from build123d import *

# Parameters (mm, degrees)
SKETCH1_R           = 4
BOSS_EXTRUDE1_DEPTH = 15
SKETCH2_R           = 6
BOSS_EXTRUDE2_DEPTH = 1
DOME1_FACE_RADIUS   = 6
DOME1_HEIGHT        = 6
SKETCH3_W           = 2
SKETCH3_H           = 12.932996947
CUT_EXTRUDE2_DEPTH  = 5


with BuildPart() as part:
    # Sketch1 → Boss-Extrude1 (new body)
    with BuildSketch(Plane.XY):
        Circle(SKETCH1_R)
    extrude(amount=BOSS_EXTRUDE1_DEPTH)

    # Sketch2 → Boss-Extrude2 (add)
    with BuildSketch(Plane.XY.offset(15)):
        Circle(SKETCH2_R)
    extrude(amount=BOSS_EXTRUDE2_DEPTH)

    # Dome1: a dome of height H over a round flat face of radius A is a cap of a sphere of radius (A * A + H * H) / (2 * H)
    dome1_r = (DOME1_FACE_RADIUS * DOME1_FACE_RADIUS + DOME1_HEIGHT * DOME1_HEIGHT) / (2 * DOME1_HEIGHT)
    dome1_base = Plane((0, 0, 16), z_dir=(0, 0, 1))
    with Locations(dome1_base.offset(DOME1_HEIGHT - dome1_r)):
        dome1_ball = Sphere(dome1_r, mode=Mode.PRIVATE)
    add(split(dome1_ball, bisect_by=dome1_base, keep=Keep.TOP, mode=Mode.PRIVATE))

    # Sketch3 → Cut-Extrude2 (cut)
    with BuildSketch(Plane.XY.offset(22)):
        with Locations((0, -0.226721745)):
            Rectangle(SKETCH3_W, SKETCH3_H)
    extrude(amount=-CUT_EXTRUDE2_DEPTH, mode=Mode.SUBTRACT)


solid = part.part
The listing builds one solid part. Answer for the finished solid, in the listing's coordinates (mm). A direction names the side the tool comes from. Give positions to 0.01 mm unless a question says otherwise; leave off trailing zeros. Write each loop counter-clockwise with the first axis right and the second up, starting at its lowest first coordinate (ties: lowest second). Pieces come first, ordered by that corner, then holes. Notation, with made-up numbers: (41, 44) -> (78, 44) arc R27 cw to (78, 61) -> close; hole circle Ø4 at (74, -8). An arc over 180 degrees is marked (long way). Use a Markdown table: item, result.
(1) Section B-B, the plane y = 0 is taken. Determine the outline of the cut face in (x, z).
Return value:
| item | result |
|---|---|
| outline | (-6, 15) -> (-4, 15) -> (-4, 0) -> (4, 0) -> (4, 15) -> (6, 15) -> (6, 16) arc R6 ccw to (1, 21.92) -> (1, 17) -> (-1, 17) -> (-1, 21.92) arc R6 ccw to (-6, 16) -> close |
(2) Section A-A, the plane x = 0 is taken. Determine the outline of the cut face in (y, z), then the cut area to 3 significant figures.
Return value:
| item | result |
|---|---|
| outline | (-6, 15) -> (-4, 15) -> (-4, 0) -> (4, 0) -> (4, 15) -> (6, 15) -> (6, 16) arc R6 ccw to (5.92, 17) -> (-5.92, 17) arc R6 ccw to (-6, 16) -> close |
| area | 144 mm2 |
(3) Flat-ended cylindrical pins translate along their axes: P1, Ø6, axis at y = -3.5, z = 17, coming from the -X side; P2, Ø6, axis at x = -1, y = 4, coming from the +Z side; P3, Ø3, axis at y = 4.5, z = 16.5, coming from the +X side. Find the tip coordinate at first contact, or state that the pin passes through.
Return value:
| item | result |
|---|---|
| P1 | x = -5.97 |
| P2 | z = 21.83 |
| P3 | x = 5.18 |
(4) Section D-D, the plane z = 14.5 is taken. Determine the outline of the cut face in (x, y), then the cut area to 3 significant figures.
Return value:
| item | result |
|---|---|
| outline | circle Ø8 at (0, 0) |
| area | 50.3 mm2 |
(5) Section C-C, the plane z = 19.5 is taken. Determine the outline of the cut face in (x, y), then the cut area to 3 significant figures.
Return value:
| item | result |
|---|---|
| outline | (-1, -4.77) -> (-1, 4.77) arc R4.87 ccw to start; (1, -4.77) arc R4.87 ccw to (1, 4.77) -> close |
| area | 55.3 mm2 |
(6) Find the intervals of material crossed by probe 1 along X at (y, z) = (5, 17.25); probe 2 along Z at (x, y) = (0.75, 1.25); probe 3 along X at (y, z) = (-1.5, 19.25), in increasing order. Write a range as from..to.
Return value:
| item | result |
|---|---|
| probe 1 | -3.07..-1, 1..3.07 |
| probe 2 | 0..17 |
| probe 3 | -4.82..-1, 1..4.82 |
(7) For faces 1 (the cylindrical face through (-0.867, -3.905, 7.395)), 2 (the flat face through (0, 0, 0)), 3 (the flat face through (0, 0, 17)), determine the directions among +Z, -Z, +X, -X, +Y, -Y from which every point of the face is accessible in a straight line to the end or side of a thin tool.
Return value:
| item | result |
|---|---|
| face 1 | -Z |
| face 2 | -Z, +X, -X, +Y, -Y |
| face 3 | +Z, +Y, -Y |
(8) Determine the mould class of faces 4 (the flat face through (-1, 0, 19)), 5 (the flat face through (-1.42, -3.92, 15)), 6 (the cylindrical face through (-5.994, 0.264, 15.493)) for opening direction X: released by +X, released by -X, zero draft, split by the parting line, or undercut.
Return value:
| item | result |
|---|---|
| face 4 | undercut |
| face 5 | zero draft |
| face 6 | split by the parting line |
